Build history of the part. All positions in model axes, mm. A direction names the side the tool comes from. Give positions to 0.01 mm unless a question says otherwise; leave off trailing zeros. Loops run counter-clockwise (first coordinate to the right, second up) from the corner with the lowest first, then second, coordinate; pieces in that order, holes last. Notation, with made-up numbers: (2.25, 85) -> (46.25, 85) arc R10 cw to (46.25, 94) -> close; hole circle Ø10 at (54.5, 58.5). An arc over 180 degrees is marked (long way). Answer in a Markdown table with one row per item. Add a question column.
from build123d import *

# Parameters (mm, degrees)
F2_R          = 60.96
F3_DEPTH      = 114.301
F3_DEPTH_BACK = 114.301
F4_W          = 259.588
F4_H          = 37.084
F5_DEPTH      = 114.301
F5_DEPTH_BACK = 114.301


with BuildPart() as f1:
    # F0 (on Front) → F1 (revolve)
    with BuildSketch(Plane.XZ):
        with BuildLine():
            Line((0, 114.3), (0, -114.3))
            ThreePointArc((0, -114.3), (114.3, 0), (0, 114.3))
        make_face()
    revolve(axis=Axis((0, 0, 0), (0, 0, -1)))

    # F2 (on Top) → F3 (cut, two sides)
    with BuildSketch(Plane.XY) as f3_sk:
        Circle(F2_R)
    extrude(amount=-F3_DEPTH, mode=Mode.SUBTRACT)
    extrude(f3_sk.sketch, amount=F3_DEPTH_BACK, mode=Mode.SUBTRACT)

    # F4 (on Front) → F5 (cut, two sides)
    with BuildSketch(Plane.XZ) as f5_sk:
        with Locations((0, 111.252)):
            Rectangle(F4_W, F4_H)
        with Locations((0, -111.252)):
            Rectangle(F4_W, F4_H)
    extrude(amount=-F5_DEPTH, mode=Mode.SUBTRACT)
    extrude(f5_sk.sketch, amount=F5_DEPTH_BACK, mode=Mode.SUBTRACT)

    # F6 (on Right) → F7 (revolve, cut)
    with BuildSketch(Plane.YZ):
        with BuildLine():
            Line((0, 67.31), (-76.1046903942, 67.31))
            ThreePointArc((-76.1046903942, 67.31), (-101.6, 0), (-76.1046903942, -67.31))
            Line((-76.1046903942, -67.31), (0, -67.31))
            Line((0, -67.31), (0, 67.31))
        make_face()
    revolve(axis=Axis((0, 0, 0), (0, 0, 1)), mode=Mode.SUBTRACT)


solid = f1.part
(1) 3-axis set-ups, long thin cutter, end or side, ignore diameter. For faces 1 (the flat face through (23, 57, -67.31)), 2 (the cylindrical face through (-13.21, -59.51, 80.19)): which of +Z, -Z, +X, -X, +Y, -Y reach the whole face in a straight line?
(2) Saw through at D-D, the plane y = 94.5. List the corners of the cut face in (x, z), then the cut area to 3 significant figures.
(3) Saw through at A-A, the plane y = 0. List the corners of the cut face in (x, z), then the cut area to 3 significant figures.
(4) Wall check: line 1 along Y through (x, z) = (0, 87.5); line 2 along X through (y, z) = (82, 46.5); line 3 along Y through (x, z) = (-64, 23.5). Give the ranges that are in metal, low to high. Write a range as from..to.
(5) Saw through at C-C, the plane z = 16. List the corners of the cut face in (x, y), then the cut area to 3 significant figures.
(6) Flat gauge pins, fed straight in: pin 1 Ø2 at (y, z) = (67.5, -38.5) entering from -X; pin 2 Ø6 at (y, z) = (55, 44.5) entering from +X; pin 3 Ø3 at (x, y) = (-21.5, 74.5) entering from -Z. Where does each tip first touch, or does it go through?
(7) Two-plate mould, pull along Z, no slides. Class faces 3 (the flat face through (29, 54, -92.71)), 4 (the flat face through (23, -57, 67.31)), 5 (the cylindrical face through (-13.21, -59.51, -79.83)), 6 (the flat face through (29, -54, 92.71)): released by +Z, released by -Z, zero draft, split by the parting line, or undercut.
Worked answers:
| question | item | result |
|---|---|---|
| 1 | face 1 | none |
| 1 | face 2 | +Z, -Z |
| 2 | outline | circle Ø128.6 at (0, 0); hole circle Ø74.63 at (0, 0) |
| 2 | area | 8,610 mm^2 |
| 3 | outline | (-76.1, -67.31) arc R101.6 cw to (-76.1, 67.31) -> (-60.96, 67.31) -> (-60.96, 92.71) -> (-66.85, 92.71) arc R114.3 ccw to (-66.85, -92.71) -> (-60.96, -92.71) -> (-60.96, -67.31) -> close; (60.96, -92.71) -> (66.85, -92.71) arc R114.3 ccw to (66.85, 92.71) -> (60.96, 92.71) -> (60.96, 67.31) -> (76.1, 67.31) arc R101.6 cw to (76.1, -67.31) -> (60.96, -67.31) -> close |
| 3 | area | 5,730 mm^2 |
| 4 | line 1 | -73.54..-60.96, 60.96..73.54 |
| 4 | line 2 | -64.64..-37.9, 37.9..64.64 |
| 4 | line 3 | -91.74..-75.33, 75.33..91.74 |
| 5 | outline | circle Ø226.35 at (0, 0); hole circle Ø200.66 at (0, 0) |
| 5 | area | 8,610 mm^2 |
| 6 | pin 1 | x = -84.74 |
| 6 | pin 2 | x = 92.06 |
| 6 | pin 3 | z = -85.34 |
| 7 | face 3 | released by -Z |
| 7 | face 4 | undercut |
| 7 | face 5 | zero draft |
| 7 | face 6 | released by +Z |
